Build history of the part. All positions in model axes, mm. Round coordinates to 2 decimals unless told otherwise and drop trailing zeros. Write each loop counter-clockwise with the first axis right and the second up, starting at its lowest first coordinate (ties: lowest second). Pieces come first, ordered by that corner, then holes. Notation, with made-up numbers: (16, 64.5) -> (60, 64.5) arc R22 ccw to (60, 87.5) -> close; hole circle Ø8 at (73, 57). An arc over 180 degrees is marked (long way). Answer as CSV lines item,"result".
from build123d import *

# Parameters (mm, degrees)
F0_W      = 400
F0_H      = 200
F1_DEPTH  = 25
F2_W      = 26.7749875784
F2_H      = 200.0415027142
F3_DEPTH  = 45
F4_W      = 163.5136380792
F4_H      = 32.6408185065
F5_DEPTH  = 400.001
F8_DEPTH  = 25
F8_TAPER  = -60
F9_W      = 212.9299342632
F9_H      = 224.1696352139
F10_DEPTH = 25
F12_W     = 417.4379836768
F12_H     = 216.8577280827
F13_DEPTH = 25


with BuildPart() as f1:
    # F0 (on Top) → F1 (new body)
    with BuildSketch(Plane.XY):
        with Locations((200, 100)):
            Rectangle(F0_W, F0_H)
    extrude(amount=-F1_DEPTH)

    # F2 (on Top) → F3 (join)
    with BuildSketch(Plane.XY):
        with Locations((203.9749994874, 100.0207513571)):
            Rectangle(F2_W, F2_H)
    extrude(amount=F3_DEPTH)

    # F4 (on Right) → F5 (cut, through all)
    with BuildSketch(Plane.YZ):
        with Locations((99.4616560638, 16.3204092532)):
            Rectangle(F4_W, F4_H)
    extrude(amount=F5_DEPTH, mode=Mode.SUBTRACT)

    # F7 (on offset) → F8 (cut)
    with BuildSketch(Plane.XY.offset(-20)):
        with BuildLine():
            add(Edge.make_bspline(
                [(391.8431701423, 100.8600369096), (391.8431701423, 259.7252513864), (102.5679333925, 180.292644148), (-186.7073033574, 100.8600369096), (102.5679333925, 21.4274296712), (391.8431701423, -58.0051775672), (391.8431701423, 100.8600369096)],
                knots=[0, 0, 0, 2.0943951024, 2.0943951024, 4.1887902048, 4.1887902048, 6.2831853072, 6.2831853072, 6.2831853072], degree=2, weights=[1, 0.5, 1, 0.5, 1, 0.5, 1]))
        make_face()
    extrude(amount=-F8_DEPTH, taper=F8_TAPER, mode=Mode.SUBTRACT)

    # F9 (on offset) → F10 (cut)
    with BuildSketch(Plane.XY.offset(-20)):
        with Locations((308.3530813456, 101.8974217586)):
            Rectangle(F9_W, F9_H)
    extrude(amount=-F10_DEPTH, mode=Mode.SUBTRACT)

    # F12 (on offset) → F13 (cut)
    with BuildSketch(Plane.XY.offset(-20)):
        with Locations((200.3057235852, 101.122589549)):
            Rectangle(F12_W, F12_H)
    extrude(amount=-F13_DEPTH, mode=Mode.SUBTRACT)


solid = f1.part
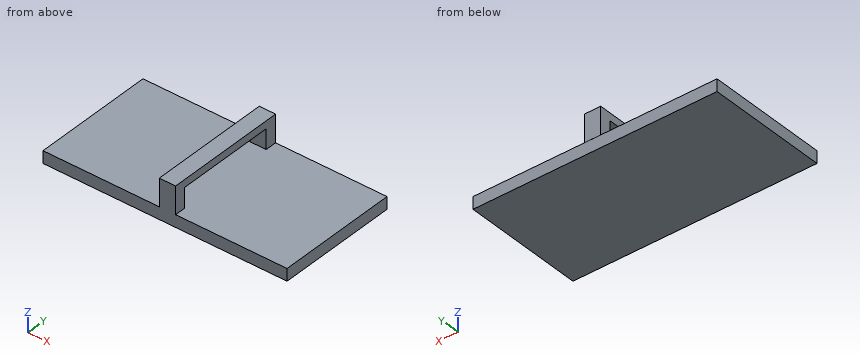
1. Cut at B-B, the plane z = 12. Write the cut outline in (x, y), then the cut area to 3 significant figures.
Results found:
outline,"(190.59, 0) -> (217.36, 0) -> (217.36, 17.7) -> (190.59, 17.7) -> close; (190.59, 181.22) -> (217.36, 181.22) -> (217.36, 200.04) -> (190.59, 200.04) -> close"
area,"978 mm2"
2. Cut at D-D, the plane z = 39.5. Write the cut outline in (x, y).
Results found:
outline,"(190.59, 0) -> (217.36, 0) -> (217.36, 200.04) -> (190.59, 200.04) -> close"
3. Cut at A-A, the plane y = 64.5. Write the cut outline in (x, z).
Results found:
outline,"(0, -20) -> (400, -20) -> (400, 0) -> (0, 0) -> close; (190.59, 32.64) -> (217.36, 32.64) -> (217.36, 45) -> (190.59, 45) -> close"
4. Cut at C-C, the plane x = 45.5. Write the cut outline in (y, z).
Results found:
outline,"(0, -20) -> (200, -20) -> (200, 0) -> (0, 0) -> close"
5. Probe line 1 along Z through (x, y) = (234.5, 162); line 2 along Y through (x, z) = (338, -9.5); line 3 along X through (y, z) = (10.5, 27.5). List the from-to ranges inside material, lowest first.
Results found:
line 1,"z = -20 to 0"
line 2,"y = 0 to 200"
line 3,"x = 190.59 to 217.36"
6. Drop flat-ended pins along their axis: pin 1 Ø22.5 at (y, z) = (96.5, 28.5) entering from +X; pin 2 Ø16 at (x, z) = (157.5, -15) entering from +Y. Give the stop position or say it passes through.
Results found:
pin 1,"stops at x = 217.36"
pin 2,"stops at y = 200"
